Autodesk Inventor part; units mm, degrees
ref_plane "YZ Plane" through (0, 0, 0) normal (1, 0, 0) x (0, 1, 0)
ref_plane "XZ Plane" through (0, 0, 0) normal (0, 1, 0) x (-1, 0, 0)
ref_plane "XY Plane" through (0, 0, 0) normal (0, 0, 1) x (1, 0, 0)
sketch "スケッチ1" plane through (0, 0, 0) normal (0, 0, 1) x (1, 0, 0)
  circle A0 centre (0, 0) radius 47.5
  circle A1 centre (0, 0) radius 67.5
  dimension "d0" = 95
  dimension "d1" = 135
extrude "押し出し1" add sketch "スケッチ1" along normal blind 20
sketch "スケッチ2" plane through (0, 0, 20) normal (0, 0, 1) x (1, 0, 0)
  circle A0 centre (0, 0) radius 62.5
  point P0 (16.1762, 60.3704)
  point P1 (-16.1762, 60.3704)
  point P2 (-44.1942, 44.1942)
  point P3 (-60.3704, 16.1762)
  point P4 (-60.3704, -16.1762)
  point P5 (-44.1942, -44.1942)
  point P6 (-16.1762, -60.3704)
  point P7 (16.1762, -60.3704)
  point P8 (44.1942, -44.1942)
  point P9 (60.3704, -16.1762)
  point P10 (60.3704, 16.1762)
  point P11 (44.1942, 44.1942)
  dimension "d4" = 125
  dimension "d7" = 360
  dimension "d25" = 0
hole "穴1" at (16.1762, 60.3704, 20) at (-16.1762, 60.3704, 20) at (-44.1942, 44.1942, 20) at (-60.3704, 16.1762, 20) at (-60.3704, -16.1762, 20) at (-44.1942, -44.1942, 20) at (-16.1762, -60.3704, 20) at (16.1762, -60.3704, 20) at (44.1942, -44.1942, 20) at (60.3704, -16.1762, 20) at (60.3704, 16.1762, 20) at (44.1942, 44.1942, 20) direction (0, 0, -1) diameter 4.5 end through all
chamfer "面取り1" distance 1 angle 45 2 edges at (-47.5, 0, 20) (-47.5, 0, 0)
sketch "スケッチ3" plane through (0, 0, 20) normal (0, 0, 1) x (1, 0, 0)
  circle A0 centre (16.1762, 60.3704) radius 2.25
  circle A1 centre (-16.1762, 60.3704) radius 2.25
  circle A2 centre (0, 0) radius 67.5
  circle A3 centre (-16.1762, 60.3704) radius 5
  circle A4 centre (16.1762, 60.3704) radius 5
  circle A5 centre (0, 0) radius 62.5
  point P0 (-11.2987, 61.4702)
  point P1 (11.2987, 61.4702)
  point P2 (17.4703, 65.2)
  point P3 (-17.4703, 65.2)
properties part number "unit-base3" material "ABS プラスチック"
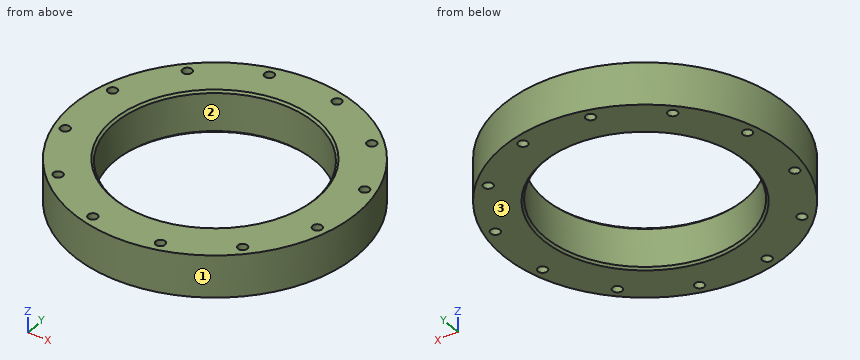
Build history of the part. All positions in model axes, mm. Face numbers are marked on the shaded views. Round coordinates to 2 decimals unless told otherwise and drop trailing zeros. Write each loop counter-clockwise with the first axis right and the second up, starting at its lowest first coordinate (ties: lowest second). Pieces come first, ordered by that corner, then holes. Notation, with made-up numbers: (48.5, 78) -> (61.5, 78) arc R8 cw to (61.5, 86) -> close; hole circle Ø11 at (7.5, 2.25). An arc over 180 degrees is marked (long way). Put each result on its own line as item: value.
Item 1: Flat gauge pins, fed straight in: P1, Ø10, axis at x = -42.5, z = 4, coming from the +Y side; P2, Ø1, axis at x = 10.5, z = 6, coming from the +Y side; P3, Ø3.5, axis at x = 16.18, y = -60.37, coming from the -Z side; P4, Ø12, axis at x = 50, z = 12.5, coming from the -Y side. Where does each tip first touch, or does it go through?
Here are the results:
P1: stops at y = 56.12
P2: stops at y = 66.76
P3: passes through
P4: stops at y = -51.19
Item 2: Wall check: probe 1 along Y at (x, z) = (16, 5.5); probe 2 along X at (y, z) = (-58.5, 18); probe 3 along Y at (x, z) = (40, 14.25). Give the ranges that are in metal, low to high. Write a range as from..to.
Here are the results:
probe 1: y = -65.58..-62.61, -58.13..-44.72, 44.72..58.13, 62.61..65.58
probe 2: x = -33.67..-17.43, -14.93..14.93, 17.43..33.67
probe 3: y = -54.37..-25.62, 25.62..54.37
Item 3: Slice it at D-D, the plane y = 55.5. Give the cut face in (x, z).
Here are the results:
outline: (-38.42, 0) -> (38.42, 0) -> (38.42, 20) -> (-38.42, 20) -> close
Item 4: Slice it at A-A, the plane y = 0. Give the cut face in (x, z).
Here are the results:
outline: (-67.5, 0) -> (-48.5, 0) -> (-47.5, 1) -> (-47.5, 19) -> (-48.5, 20) -> (-67.5, 20) -> close; (47.5, 1) -> (48.5, 0) -> (67.5, 0) -> (67.5, 20) -> (48.5, 20) -> (47.5, 19) -> close
Item 5: Slice it at C-C, the plane z = 5.5. Count the separate pieces of the cut face and the enclosed holes in it, plus the area to 3 significant figures.
Here are the results:
separate pieces: 1
enclosed holes: 13
area: 7,030 mm^2
Item 6: Two-plate mould, pull along X, no slides. Class the marked faces 1, 2 and 3: pulls with the +X half, pulls with the -X half, needs draft (parallel to the pull), parting line crosses it, or undercut.
Here are the results:
face 1: parting line crosses it
face 2: undercut
face 3: needs draft
